Source: CAD feature listing. Evaluate the final solid. Frame: model axes, mm. A direction names the side the tool comes from. Give positions to 0.01 mm unless a question says otherwise; leave off trailing zeros. Order: outer loops, then holes, each group sorted by start corner. A loop starts at its lowest first (then second) coordinate and runs counter-clockwise, first axis right, second up.
1) Material intervals for line 1 (X direction, y = 5.5, z = -83); line 2 (Y direction, x = 21, z = -32); line 3 (Z direction, x = 47.5, y = 83), sorted ascending.
2) Section C-C, the plane y = 20. Return loops of the section in (x, z), plus the area to 3 significant figures.
3) Section B-B, the plane z = -50. Return loops of the section in (x, y), plus the area to 3 significant figures.
4) Access query for faces 1 (the face through (30, 32, 0)), 2 (the face through (42, 42, -100)), 3 (the face through (13, 40, -49)), 4 (the face through (70, 52, -65)), 5 (the face through (60, 42, -30)). Directions: +Z, -Z, +X, -X, +Y, -Y. A direction counts if a zero-diameter tool reaches every point of the face in a straight line with its end or side. Return the directions, or none.
5) Section A-A, the plane y = 74. Return loops of the section in (x, z).
6) Section D-D, the plane x = -17. Return loops of the section in (y, z), plus the area to 3 significant figures.
7) First-contact query: P1, Ø21, axis at y = 29, z = -57.5, coming from the +X side; P2, Ø10.5, axis at x = 52.5, y = 90.5, coming from the +Z side; P3, Ø18, axis at y = 72.5, z = -85.5, coming from the -X side; P4, Ø1, axis at x = 38, z = -126.5, coming from the -Y side. Flat tips, straight axial feed; report the tip coordinate or a pass-through.
```python
from build123d import *

# Parameters (mm, degrees)
EXTRUDE1_DEPTH = 100
SKETCH2_W      = 35
SKETCH2_H      = 30
EXTRUDE2_DEPTH = 105
SKETCH3_W      = 20
SKETCH3_H      = 30
EXTRUDE3_DEPTH = 105
EXTRUDE4_DEPTH = 31
SKETCH5_R      = 110
EXTRUDE5_DEPTH = 0.1


with BuildPart() as part:
    # Sketch1 → Extrude1 (new body)
    with BuildSketch(Plane.XY):
        with BuildLine():
            Line((0, 0), (70, 0))
            Line((70, 0), (70, 85))
            ThreePointArc((70, 85), (38.180194847, 71.819805153), (25, 40))
            Line((25, 40), (0, 40))
            Line((0, 40), (0, 0))
        make_face()
    extrude(amount=-EXTRUDE1_DEPTH)

    # Sketch2 → Extrude2 (add)
    with BuildSketch(Plane(origin=(0, 0, 0), x_dir=(1, 0, 0), z_dir=(0, 1, 0))):
        with Locations((52.5, 85)):
            Rectangle(SKETCH2_W, SKETCH2_H)
    extrude(amount=EXTRUDE2_DEPTH)

    # Sketch3 → Extrude3 (cut)
    with BuildSketch(Plane(origin=(0, 0, 0), x_dir=(1, 0, 0), z_dir=(0, 1, 0))):
        with Locations((60, 15)):
            Rectangle(SKETCH3_W, SKETCH3_H)
    extrude(amount=EXTRUDE3_DEPTH, mode=Mode.SUBTRACT)

    # Sketch4 → Extrude4 (cut, through all)
    with BuildSketch(Plane.XY.offset(-70)):
        Polygon((70, 105), (35, 105), (35, 84.792740578), align=None)
    extrude(amount=-EXTRUDE4_DEPTH, mode=Mode.SUBTRACT)

    # Sketch5 → Extrude5 (add)
    with BuildSketch(Plane(origin=(0, 0, 0), x_dir=(1, 0, 0), z_dir=(0, 1, 0))):
        with Locations(Location((35, 50, 0), (0, 0, 270))):  # turned: the seam where the file's is
            Circle(SKETCH5_R)
    extrude(amount=EXTRUDE5_DEPTH)


solid = part.part
```
From the geometry:
1. line 1: x = 0 to 70
1. line 2: y = 0 to 40
1. line 3: z = -100 to -70
2. outline: (0, -100) - (70, -100) - (70, -30) - (50, -30) - (50, 0) - (0, 0) - close
2. area: 6,400 mm2
3. outline: (-75, 0) - (145, 0) - (145, 0.1) - (70, 0.1) - (70, 85) arc R45 ccw to (25, 40) - (0, 40) - (0, 0.1) - (-75, 0.1) - close
3. area: 4,410 mm2
4. face 1: +Z, +X, -X, +Y
4. face 2: -Z, +X, -X, +Y
4. face 3: +Z, -Z, -X, +Y
4. face 4: +Z, -Z, +X, +Y
4. face 5: +Z, +X, +Y
5. outline: (35, -100) - (70, -100) - (70, -30) - (50, -30) - (50, 0) - (40.52, 0) - (40.52, -70) - (35, -70) - close
6. outline: (0, -146.93) - (0.1, -146.93) - (0.1, 46.93) - (0, 46.93) - close
6. area: 19.4 mm2
7. P1: stops at x = 70
7. P2: stops at z = -70
7. P3: stops at x = 31.62
7. P4: stops at y = 0
